```python
from build123d import *

# Parameters (mm, degrees)
SKETCH1_R                                       = 4
SKETCH1_R_2                                     = 2.5
BOSS_EXTRUDE1_DEPTH                             = 7.9375
SKETCH3_R                                       = 12.5
SKETCH3_R_2                                     = 4
BOSS_EXTRUDE2_DEPTH                             = 5
CUT_EXTRUDE1_START                              = -2.5
SKETCH4_R                                       = 12.5
SKETCH4_R_2                                     = 6
CUT_EXTRUDE1_DEPTH                              = 2.5
CHAMFER1_SIZE                                   = 10
CUT_EXTRUDE2_START                              = -1.5
SKETCH5_R                                       = 6
CUT_EXTRUDE2_DEPTH                              = 1.5
CSK_FOR_M5_OVAL_HEAD_MACHINE_SCREW2_D           = 5.8
CSK_FOR_M5_OVAL_HEAD_MACHINE_SCREW2_CSINK_D     = 10.4
CSK_FOR_M5_OVAL_HEAD_MACHINE_SCREW2_CSINK_ANGLE = 90
CSK_FOR_M5_OVAL_HEAD_MACHINE_SCREW3_D           = 5.8
CSK_FOR_M5_OVAL_HEAD_MACHINE_SCREW3_CSINK_D     = 10.4
CSK_FOR_M5_OVAL_HEAD_MACHINE_SCREW3_CSINK_ANGLE = 90


with BuildPart() as part:
    # Sketch1 → Boss-Extrude1 (new body)
    with BuildSketch(Plane.XY):
        with BuildLine():
            Line((-45, 0), (-45, -65.863068229))
            Line((-45, -65.863068229), (-45, -72.736931771))
            Line((-45, -72.736931771), (-45, -165.863068229))
            Line((-45, -165.863068229), (-45, -172.736931771))
            Line((-45, -172.736931771), (-45, -219.3))
            Line((-45, -219.3), (-38.7, -219.3))
            Line((-38.7, -219.3), (-38.7, -269.3))
            ThreePointArc((-38.7, -269.3), (0, -308), (38.7, -269.3))
            Line((38.7, -269.3), (38.7, -219.3))
            Line((38.7, -219.3), (45, -219.3))
            Line((45, -219.3), (45, -172.736931771))
            Line((45, -172.736931771), (45, -165.863068229))
            Line((45, -165.863068229), (45, -72.736931771))
            Line((45, -72.736931771), (45, -65.863068229))
            Line((45, -65.863068229), (45, 0))
            ThreePointArc((45, 0), (0, 45), (-45, 0))
        make_face()
        with Locations((0, -269.3)):
            Circle(SKETCH1_R, mode=Mode.SUBTRACT)
        with Locations((0, -89.3)):
            Circle(SKETCH1_R_2, mode=Mode.SUBTRACT)
        with Locations((0, -149.3)):
            Circle(SKETCH1_R_2, mode=Mode.SUBTRACT)
        with Locations((20, -149.3)):
            Circle(SKETCH1_R_2, mode=Mode.SUBTRACT)
        with Locations(Location((-20, -149.3, 0), (0, 0, 180))):
            Circle(SKETCH1_R_2, mode=Mode.SUBTRACT)
        with Locations((-40, -49.3)):
            Circle(SKETCH1_R_2, mode=Mode.SUBTRACT)
        with Locations((-40, -169.3)):
            Circle(SKETCH1_R_2, mode=Mode.SUBTRACT)
        with Locations(Location((40, -169.3, 0), (0, 0, 180))):
            Circle(SKETCH1_R_2, mode=Mode.SUBTRACT)
        with Locations(Location((40, -49.3, 0), (0, 0, 180))):
            Circle(SKETCH1_R_2, mode=Mode.SUBTRACT)
        with Locations((-22.943057454, 32.766081772)):
            Circle(SKETCH1_R_2, mode=Mode.SUBTRACT)
        with Locations((22.943057454, 32.766081772)):
            Circle(SKETCH1_R_2, mode=Mode.SUBTRACT)
        with Locations((-40, -94.3)):
            Circle(SKETCH1_R_2, mode=Mode.SUBTRACT)
    extrude(amount=BOSS_EXTRUDE1_DEPTH)

    # Sketch3 → Boss-Extrude2 (add)
    with BuildSketch(Plane.XY.offset(7.9375)):
        with Locations(Location((0, -269.3, 0), (0, 0, 180))):
            Circle(SKETCH3_R)
        with Locations((0, -269.3)):
            Circle(SKETCH3_R_2, mode=Mode.SUBTRACT)
    extrude(amount=BOSS_EXTRUDE2_DEPTH)

    # Sketch4 → Cut-Extrude1 (cut)
    with BuildSketch(Plane.XY.offset(12.9375).offset(CUT_EXTRUDE1_START)):
        with Locations(Location((0, -269.3, 0), (0, 0, 180))):
            Circle(SKETCH4_R)
        with Locations((0, -269.3)):
            Circle(SKETCH4_R_2, mode=Mode.SUBTRACT)
    extrude(amount=CUT_EXTRUDE1_DEPTH, mode=Mode.SUBTRACT)

    # Chamfer1
    # the kernel refuses this chamfer: 10 mm, written as the material it takes off along each edge
    with BuildSketch(Plane(origin=(45, -219.3, -25.71682988), x_dir=(0.027495876610586282, 0.9996219169112968, 0), z_dir=(0, 0, 1))) as chamfer1_piece_1_section:
        Polygon((CHAMFER1_SIZE * 0.999621916911, CHAMFER1_SIZE * 0.0274958766106), (-CHAMFER1_SIZE * 0.0274958766106, CHAMFER1_SIZE * 0.999621916911), (0, 0), align=None)
    chamfer1_piece_1 = extrude(amount=59.371159759, mode=Mode.PRIVATE)
    chamfer1_piece_1 = split(chamfer1_piece_1, bisect_by=Plane(origin=(38.7, -215.600664049, 3.96875), z_dir=(1, 0, 0)), keep=Keep.TOP, mode=Mode.PRIVATE)
    add(chamfer1_piece_1, mode=Mode.SUBTRACT)
    with BuildSketch(Plane(origin=(-45, -219.3, -25.71682988), x_dir=(-0.027495876610586282, 0.9996219169112968, 0), z_dir=(0, 0, 1))) as chamfer1_piece_2_section:
        Polygon((CHAMFER1_SIZE * 0.999621916911, -CHAMFER1_SIZE * 0.0274958766106), (-CHAMFER1_SIZE * 0.0274958766106, -CHAMFER1_SIZE * 0.999621916911), (0, 0), align=None)
    chamfer1_piece_2 = extrude(amount=59.371159759, mode=Mode.PRIVATE)
    chamfer1_piece_2 = split(chamfer1_piece_2, bisect_by=Plane(origin=(-38.7, -215.600664049, 3.96875), z_dir=(-1, 0, 0)), keep=Keep.TOP, mode=Mode.PRIVATE)
    add(chamfer1_piece_2, mode=Mode.SUBTRACT)

    # Sketch5 → Cut-Extrude2 (cut)
    with BuildSketch(Plane.XY.offset(12.9375).offset(CUT_EXTRUDE2_START)):
        with Locations((0, -269.3)):
            Circle(SKETCH5_R)
    extrude(amount=CUT_EXTRUDE2_DEPTH, mode=Mode.SUBTRACT)

    # CSK for M5 Oval Head Machine Screw2 (through all)
    with Locations(Plane(origin=(40, -49.3, 0), x_dir=(-1, 0, 0), z_dir=(0, 0, -1))):
        with Locations((0, 0), (40, -40), (80, 0), (80, -120), (60, -100), (40, -100), (20, -100), (0, -120)):
            CounterSinkHole(CSK_FOR_M5_OVAL_HEAD_MACHINE_SCREW2_D / 2, CSK_FOR_M5_OVAL_HEAD_MACHINE_SCREW2_CSINK_D / 2, counter_sink_angle=CSK_FOR_M5_OVAL_HEAD_MACHINE_SCREW2_CSINK_ANGLE)

    # CSK for M5 Oval Head Machine Screw3 (through all)
    with Locations(Plane(origin=(22.943057454, 32.766081772, 0), x_dir=(-1, 0, 0), z_dir=(0, 0, -1))):
        with Locations((0, 0), (45.886114908, 0)):
            CounterSinkHole(CSK_FOR_M5_OVAL_HEAD_MACHINE_SCREW3_D / 2, CSK_FOR_M5_OVAL_HEAD_MACHINE_SCREW3_CSINK_D / 2, counter_sink_angle=CSK_FOR_M5_OVAL_HEAD_MACHINE_SCREW3_CSINK_ANGLE)


solid = part.part
```
Check sheet for the modelled part. Datum: model origin and axes. Units: mm. A direction names the side the tool comes from. Round coordinates to 2 decimals unless told otherwise and drop trailing zeros. Write each loop counter-clockwise with the first axis right and the second up, starting at its lowest first coordinate (ties: lowest second). Pieces come first, ordered by that corner, then holes. Notation, with made-up numbers: M -7.5,-10 L 3.5,-10 A12 ccw 3.5,3 Z; hole C 34.25,51.5 d5. An arc over 180 degrees is marked long. Write item = value, one per line. Start each with the question number.
1. Release check for a two-part mould opening along X. For faces 3 (the flat face through (-38.7, -242, 4)), 4 (the cylindrical face through (22.314, 29.935, 5.158)), 5 (the flat face through (38.7, -243, 4)), 6 (the flat face through (-1, -129, 7.938)) record: pulls with the +X half, pulls with the -X half, needs draft (parallel to the pull), parting line crosses it, or undercut.
2. Scan lines: line 1 (Y direction, x = 0, z = 5.1); line 2 (Y direction, x = 40, z = 5.6); line 3 (Z direction, x = -2.5, y = -254.5). Record each from-to range of solid material in increasing order. Write a range as [from, to].
3. Section check B-B, the plane y = -119.5. Record the cut outline in (x, z).
4. Tool access check on faces 1 (the cylindrical face through (-38.66, -171.87, 5.16)), 2 (the cylindrical face through (2.769, -274.623, 10.93)). Record the directions out of +Z, -Z, +X, -X, +Y, -Y that give a thin tool (end or side, any length) a straight path to the whole face; none if there is none.
5. Section check A-A, the plane z = 4.5. State how many separate pieces and enclosed holes the cut face has, then the cut area to 3 significant figures.
6. Gauge pin test, flat ends, axial feed: pin 1 (4 mm diameter, centred on y = -220, z = 9.5, fed in from -X); pin 2 (7.5 mm diameter, centred on x = 0, y = -89.3, fed in from -Z); pin 3 (2 mm diameter, centred on x = -30, z = 5.5, fed in from -Y). Record the tip position at first contact, or that the pin passes through.
7. Section check C-C, the plane y = -229. Record the cut outline in (x, z).
Results found:
q1.face_3 = pulls with the -X half
q1.face_4 = undercut
q1.face_5 = pulls with the +X half
q1.face_6 = needs draft
q2.line_1 = [-308, -273.3], [-265.3, -152.2], [-146.4, -92.2], [-86.4, 45]
q2.line_2 = [-214.3, -172.2], [-166.4, -52.2], [-46.4, 20.62]
q2.line_3 = [0, 7.94]
q3.outline = M -45,0 L 45,0 L 45,7.94 L -45,7.94 Z
q4.face_1 = +Z, -Z
q4.face_2 = +Z
q5.separate_pieces = 1
q5.enclosed_holes = 12
q5.area = 28,700 mm^2
q6.pin_1 = -38.7
q6.pin_2 = 1.45
q6.pin_3 = -294.93
q7.outline = M -38.7,0 L 38.7,0 L 38.7,7.94 L -38.7,7.94 Z
